Can you work these out from the model? Positions are in its coordinate system, mm. Round coordinates to 2 decimals unless told otherwise and drop trailing zeros. Loops run counter-clockwise (first coordinate to the right, second up) from the corner with the lowest first, then second, coordinate; pieces in that order, holes last.
(1) I want a section at A-A on y = 13.5. Write out the boundary of the cut face in (x, z) (3 decimals).
(2) I want a section at C-C on x = 726. Write out the boundary of the cut face in (y, z).
(3) Will these pins go through, and if not, where does the flat tip stop? pin 1 Ø1.5 at (y, z) = (12, -68) entering from -X; pin 2 Ø12 at (y, z) = (4.5, -12.5) entering from +X (3 decimals); pin 3 Ø19 at (x, y) = (66, 22) entering from -Z.
(4) If I drill on line 1 along X through (y, z) = (16.5, -13) (3 decimals); line 2 along X through (y, z) = (29, -66); line 3 along Z through (x, y) = (796.5, 9), over which ranges is the centre line in solid material (lowest first)?
(5) I want a section at B-B on z = -63. Write out the boundary of the cut face in (x, y), plus the area to 3 significant figures.
from build123d import *

# Parameters (mm, degrees)
SKETCH1_W           = 863.6
SKETCH1_H           = 88.9
BOSS_EXTRUDE1_DEPTH = 38.1
SKETCH3_W           = 88.9
SKETCH3_H           = 38.1
CUT_EXTRUDE1_DEPTH  = 39.1
SKETCH4_W           = 180.975
SKETCH4_H           = 38.1
CUT_EXTRUDE2_DEPTH  = 39.1


with BuildPart() as part:
    # Sketch1 → Boss-Extrude1 (new body)
    with BuildSketch(Plane(origin=(0, 0, 0), x_dir=(1, 0, 0), z_dir=(0, 1, 0))):
        with Locations((431.8, 44.45)):
            Rectangle(SKETCH1_W, SKETCH1_H)
    extrude(amount=BOSS_EXTRUDE1_DEPTH)

    # Sketch3 → Cut-Extrude1 (cut, through all)
    with BuildSketch(Plane(origin=(0, 38.1, 0), x_dir=(1, 0, 0), z_dir=(0, 1, 0))):
        with Locations((44.45, 69.85)):
            Rectangle(SKETCH3_W, SKETCH3_H)
        with Locations((819.15, 69.85)):
            Rectangle(SKETCH3_W, SKETCH3_H)
    extrude(amount=-CUT_EXTRUDE1_DEPTH, mode=Mode.SUBTRACT)

    # Sketch4 → Cut-Extrude2 (cut, through all)
    with BuildSketch(Plane(origin=(0, 38.1, 0), x_dir=(1, 0, 0), z_dir=(0, 1, 0))):
        with Locations((773.1125, 19.05)):
            Rectangle(SKETCH4_W, SKETCH4_H)
    extrude(amount=-CUT_EXTRUDE2_DEPTH, mode=Mode.SUBTRACT)


solid = part.part
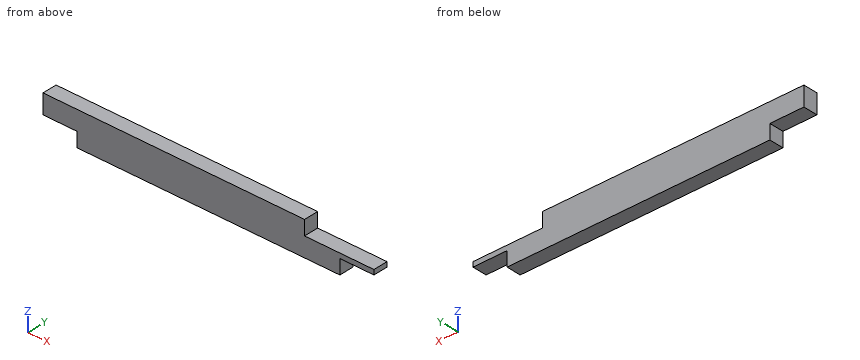
Filled sheet:
1. outline: (0, -50.8) - (88.9, -50.8) - (88.9, -88.9) - (774.7, -88.9) - (774.7, -50.8) - (863.6, -50.8) - (863.6, -38.1) - (682.625, -38.1) - (682.625, 0) - (0, 0) - close
2. outline: (0, -88.9) - (38.1, -88.9) - (38.1, -38.1) - (0, -38.1) - close
3. pin 1: stops at x = 88.9
3. pin 2: stops at x = 682.625
3. pin 3: stops at z = -50.8
4. line 1: x = 0 to 682.625
4. line 2: x = 88.9 to 774.7
4. line 3: z = -50.8 to -38.1
5. outline: (88.9, 0) - (774.7, 0) - (774.7, 38.1) - (88.9, 38.1) - close
5. area: 26,100 mm2
